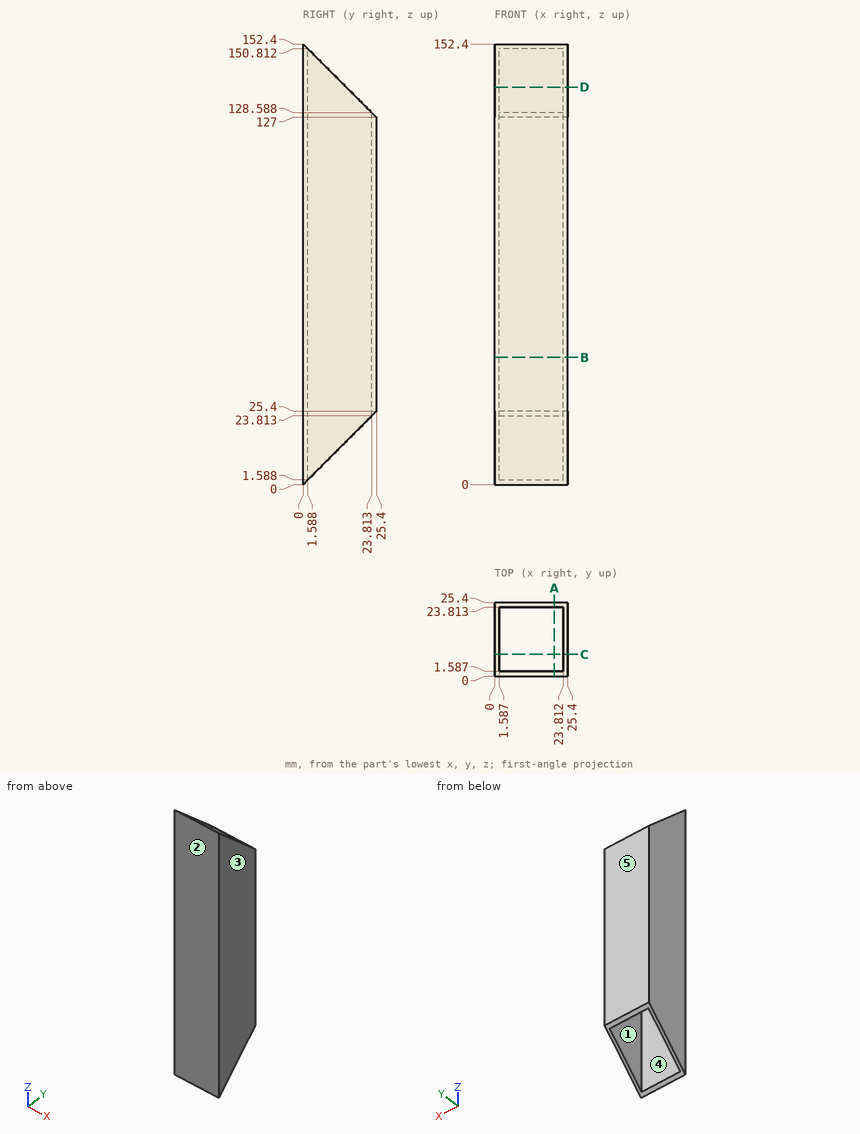
Could you check a few things on this drawing? It's one solid part, dimensions in mm from its lowest x, y, z. A direction names the side the tool comes from. Give positions to 0.01 mm unless a question says otherwise; leave off trailing zeros. Order: outer loops, then holes, each group sorted by start corner. A loop starts at its lowest first (then second) coordinate and runs counter-clockwise, first axis right, second up. Notation, with made-up numbers: (16.5, 15.5) -> (61.5, 15.5) arc R10 ccw to (61.5, 21.5) -> close; hole circle Ø3 at (-19.75, 88). An arc over 180 degrees is marked (long way). Answer in a Markdown table with one row per item. Add a question column.
Item 1: Imagine slicing it at D-D (z = 137.5). List the corners of the cut face in (x, y) for me.
Item 2: We'd pull the mould along X, two halves only. Please class the marked faces 3, 4 and 5: pulls with the +X half, pulls with the -X half, needs draft (parallel to the pull), parting line crosses it, or undercut.
Item 3: For the marked faces 1 and 2, which set-ups out of +Z, -Z, +X, -X, +Y, -Y let a thin tool reach every point of the face, with its end or its side?
Item 4: I'm going to push a flat-ended pin straight in: P1, Ø5, axis at x = 19.5, y = 20.5, coming from the +Z side. Where does the tip first touch, or does it pass through?
Item 5: Imagine slicing it at B-B (z = 44). List the corners of the cut face in (x, y) for me.
Item 6: Imagine slicing it at A-A (x = 20.75). List the corners of the cut face in (y, z) for me.
Item 7: Imagine slicing it at C-C (y = 7.5). List the corners of the cut face in (x, z) for me.
Item 8: Please list where these lines run through material, in increasing order: probe 1 along Y at (x, z) = (17, 97); probe 2 along Y at (x, z) = (13, 130).
Result:
| question | item | result |
|---|---|---|
| 1 | outline | (0, 0) -> (25.4, 0) -> (25.4, 14.9) -> (23.81, 14.9) -> (23.81, 1.59) -> (1.59, 1.59) -> (1.59, 14.9) -> (0, 14.9) -> close |
| 2 | face 3 | pulls with the +X half |
| 2 | face 4 | undercut |
| 2 | face 5 | needs draft |
| 3 | face 1 | +Z, -Z |
| 3 | face 2 | +Z, -Z, +X, -X, -Y |
| 4 | P1 | through |
| 5 | outline | (0, 0) -> (25.4, 0) -> (25.4, 25.4) -> (0, 25.4) -> close; hole (1.59, 1.59) -> (23.81, 1.59) -> (23.81, 23.81) -> (1.59, 23.81) -> close |
| 6 | outline | (0, 0) -> (1.59, 1.59) -> (1.59, 150.81) -> (0, 152.4) -> close; (23.81, 23.81) -> (25.4, 25.4) -> (25.4, 127) -> (23.81, 128.59) -> close |
| 7 | outline | (0, 7.5) -> (1.59, 7.5) -> (1.59, 144.9) -> (0, 144.9) -> close; (23.81, 7.5) -> (25.4, 7.5) -> (25.4, 144.9) -> (23.81, 144.9) -> close |
| 8 | probe 1 | 0 to 1.59, 23.81 to 25.4 |
| 8 | probe 2 | 0 to 1.59 |
